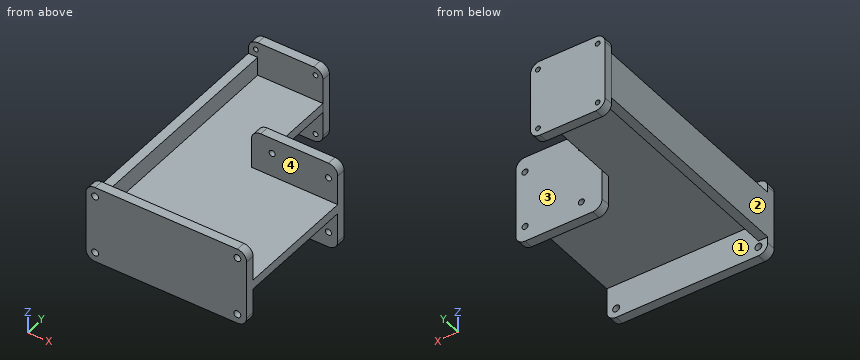
```python
from build123d import *

# Parameters (mm, degrees)
SKT_BASE_W_MOUNTING_HOLES_R           = 1.85
EXT_BASE_PLATE_W_MOUNTING_HOLES_DEPTH = 5
SKT_UPWARD_RIDGE_W                    = 86.25
SKT_UPWARD_RIDGE_H                    = 5
EXT_UPWARD_FLANGE_DEPTH               = 65
EXT_PIX_PLATFORM_DEPTH                = 5
PIX_MOUNT_HOLES_REACH                 = 91.649
SKETCH7_R                             = 1.625
SKETCH8_W                             = 40
SKETCH8_H                             = 5
GPS_FLANGE_DEPTH                      = 55
SKETCH9_R                             = 1.3
GPS_PLATFORM_DEPTH                    = 5
SKETCH10_W                            = 10
SKETCH10_H                            = 120
BRACING_DEPTH                         = 5


with BuildPart() as part:
    # Skt - Base w mounting holes → Ext - Base Plate w Mounting Holes (new body)
    with BuildSketch(Plane(origin=(0, 0, 0), x_dir=(1, 0, 0), z_dir=(0, 1, 0))):
        with BuildLine():
            Line((-38.125, 20.75), (38.125, 20.75))
            ThreePointArc((38.125, 20.75), (41.660533906, 19.285533906), (43.125, 15.75))
            Line((43.125, 15.75), (43.125, -15.75))
            ThreePointArc((43.125, -15.75), (41.660533906, -19.285533906), (38.125, -20.75))
            Line((38.125, -20.75), (-38.125, -20.75))
            ThreePointArc((-38.125, -20.75), (-41.660533906, -19.285533906), (-43.125, -15.75))
            Line((-43.125, -15.75), (-43.125, 15.75))
            ThreePointArc((-43.125, 15.75), (-41.660533906, 19.285533906), (-38.125, 20.75))
        make_face()
        with Locations(Location((-38.125, 15.75, 0), (0, 0, 270))):
            Circle(SKT_BASE_W_MOUNTING_HOLES_R, mode=Mode.SUBTRACT)
        with Locations(Location((38.125, 15.75, 0), (0, 0, 270))):
            Circle(SKT_BASE_W_MOUNTING_HOLES_R, mode=Mode.SUBTRACT)
        with Locations(Location((38.125, -15.75, 0), (0, 0, 270))):
            Circle(SKT_BASE_W_MOUNTING_HOLES_R, mode=Mode.SUBTRACT)
        with Locations(Location((-38.125, -15.75, 0), (0, 0, 270))):
            Circle(SKT_BASE_W_MOUNTING_HOLES_R, mode=Mode.SUBTRACT)
    extrude(amount=EXT_BASE_PLATE_W_MOUNTING_HOLES_DEPTH)

    # Skt - Upward Ridge → Ext - Upward Flange (add)
    with BuildSketch(Plane(origin=(0, 5, 0), x_dir=(1, 0, 0), z_dir=(0, 1, 0))):
        Rectangle(SKT_UPWARD_RIDGE_W, SKT_UPWARD_RIDGE_H)
    extrude(amount=EXT_UPWARD_FLANGE_DEPTH)

    # Skt - GPS Nest → Ext - PIX Platform (add)
    with BuildSketch(Plane(origin=(0, 70, 0), x_dir=(1, 0, 0), z_dir=(0, 1, 0))):
        with BuildLine():
            Line((1.875, 23.5), (38.125, 23.5))
            ThreePointArc((38.125, 23.5), (41.660533906, 22.035533906), (43.125, 18.5))
            Line((43.125, 18.5), (43.125, -18.5))
            ThreePointArc((43.125, -18.5), (41.660533906, -22.035533906), (38.125, -23.5))
            Line((38.125, -23.5), (1.875, -23.5))
            ThreePointArc((1.875, -23.5), (-1.660533906, -22.035533906), (-3.125, -18.5))
            Line((-3.125, -18.5), (-3.125, 18.5))
            ThreePointArc((-3.125, 18.5), (-1.660533906, 22.035533906), (1.875, 23.5))
        make_face()
    extrude(amount=EXT_PIX_PLATFORM_DEPTH)

    # Sketch7 → Pix Mount Holes (cut, up to next)
    with BuildSketch(Plane(origin=(0, 75, 0), x_dir=(1, 0, 0), z_dir=(0, 1, 0)), mode=Mode.PRIVATE) as pix_mount_holes_sk1:
        with Locations(Location((7.975, 15.25, 0), (0, 0, 270))):
            Circle(SKETCH7_R)
    pix_mount_holes_tool1 = extrude(pix_mount_holes_sk1.sketch, amount=-PIX_MOUNT_HOLES_REACH, mode=Mode.PRIVATE) & part.part
    # Sketch7 → Pix Mount Holes (cut, up to next)
    with BuildSketch(Plane(origin=(0, 75, 0), x_dir=(1, 0, 0), z_dir=(0, 1, 0)), mode=Mode.PRIVATE) as pix_mount_holes_sk2:
        with Locations(Location((38.125, 15.25, 0), (0, 0, 270))):
            Circle(SKETCH7_R)
    pix_mount_holes_tool2 = extrude(pix_mount_holes_sk2.sketch, amount=-PIX_MOUNT_HOLES_REACH, mode=Mode.PRIVATE) & part.part
    # Sketch7 → Pix Mount Holes (cut, up to next)
    with BuildSketch(Plane(origin=(0, 75, 0), x_dir=(1, 0, 0), z_dir=(0, 1, 0)), mode=Mode.PRIVATE) as pix_mount_holes_sk3:
        with Locations(Location((38.125, -15.25, 0), (0, 0, 270))):
            Circle(SKETCH7_R)
    pix_mount_holes_tool3 = extrude(pix_mount_holes_sk3.sketch, amount=-PIX_MOUNT_HOLES_REACH, mode=Mode.PRIVATE) & part.part
    # Sketch7 → Pix Mount Holes (cut, up to next)
    with BuildSketch(Plane(origin=(0, 75, 0), x_dir=(1, 0, 0), z_dir=(0, 1, 0)), mode=Mode.PRIVATE) as pix_mount_holes_sk4:
        with Locations(Location((7.975, -15.25, 0), (0, 0, 270))):
            Circle(SKETCH7_R)
    pix_mount_holes_tool4 = extrude(pix_mount_holes_sk4.sketch, amount=-PIX_MOUNT_HOLES_REACH, mode=Mode.PRIVATE) & part.part
    add(pix_mount_holes_tool1.solids().sort_by_distance((7.975, 75, -15.25))[0], mode=Mode.SUBTRACT)
    add(pix_mount_holes_tool2.solids().sort_by_distance((38.125, 75, -15.25))[0], mode=Mode.SUBTRACT)
    add(pix_mount_holes_tool3.solids().sort_by_distance((38.125, 75, 15.25))[0], mode=Mode.SUBTRACT)
    add(pix_mount_holes_tool4.solids().sort_by_distance((7.975, 75, 15.25))[0], mode=Mode.SUBTRACT)

    # Sketch8 → GPS Flange (add)
    with BuildSketch(Plane(origin=(0, 70, 0), x_dir=(1, 0, 0), z_dir=(0, 1, 0))):
        with Locations((-23.125, 0)):
            Rectangle(SKETCH8_W, SKETCH8_H)
    extrude(amount=GPS_FLANGE_DEPTH)

    # Sketch9 → GPS Platform (add)
    with BuildSketch(Plane(origin=(0, 125, 0), x_dir=(1, 0, 0), z_dir=(0, 1, 0))):
        with BuildLine():
            Line((-38.094429072, 20.75), (-8.155570928, 20.75))
            ThreePointArc((-8.155570928, 20.75), (-4.620037022, 19.285533906), (-3.155570928, 15.75))
            Line((-3.155570928, 15.75), (-3.155570928, -15.75))
            ThreePointArc((-3.155570928, -15.75), (-4.620037022, -19.285533906), (-8.155570928, -20.75))
            Line((-8.155570928, -20.75), (-38.094429072, -20.75))
            ThreePointArc((-38.094429072, -20.75), (-41.629962978, -19.285533906), (-43.094429072, -15.75))
            Line((-43.094429072, -15.75), (-43.094429072, 15.75))
            ThreePointArc((-43.094429072, 15.75), (-41.629962978, 19.285533906), (-38.094429072, 20.75))
        make_face()
        with Locations(Location((-39.125, 16.5, 0), (0, 0, 270))):
            Circle(SKETCH9_R, mode=Mode.SUBTRACT)
        with Locations(Location((-7.125, 16.5, 0), (0, 0, 270))):
            Circle(SKETCH9_R, mode=Mode.SUBTRACT)
        with Locations(Location((-7.125, -16.5, 0), (0, 0, 270))):
            Circle(SKETCH9_R, mode=Mode.SUBTRACT)
        with Locations(Location((-39.125, -16.5, 0), (0, 0, 270))):
            Circle(SKETCH9_R, mode=Mode.SUBTRACT)
    extrude(amount=GPS_PLATFORM_DEPTH)

    # Sketch10 → Bracing (add)
    with BuildSketch(Plane.ZY.offset(43.125)):
        with Locations((-7.5, 65)):
            Rectangle(SKETCH10_W, SKETCH10_H)
        with Locations((7.5, 65)):
            Rectangle(SKETCH10_W, SKETCH10_H)
    extrude(amount=-BRACING_DEPTH)


solid = part.part
```
Here's how the part is built. I have some questions about the finished solid (model axes, mm). Face numbers are marked on the shaded views. A direction names the side the tool comes from. Coordinates: 2 decimals unless noted, no trailing zeros. Order: outer loops, then holes, each group sorted by start corner. A loop starts at its lowest first (then second) coordinate and runs counter-clockwise, first axis right, second up.
1) Imagine slicing it at D-D on y = 11. List the corners of the cut face in (x, z) for me (3 decimals).
2) I need wall thicknesses on line 1 (X direction, y = 1.25, z = 15.75) (3 decimals); line 2 (Y direction, x = -8.5, z = 17); line 3 (Y direction, x = 25.5, z = -8). Which ranges of each line are inside material? Lowest first, please.
3) Imagine slicing it at C-C on x = -28. List the corners of the cut face in (y, z) for me.
4) Which directions (+Z, -Z, +X, -X, +Y, -Y) give clear straight access to the entire face, cutting with the end or side of a thin tool? Please do the marked faces 1, 2, 3 and 4.
5) Imagine slicing it at A-A on z = 6. List the corners of the cut face in (x, y) for me (3 decimals), and give its area (3 significant figures).
6) Imagine slicing it at B-B on y = 89. List the corners of the cut face in (x, z) for me (3 decimals).
7) Will these pins go through, and if not, where does the flat tip stop? pin 1 (4 mm diameter, centred on x = -28.5, y = 127.5, fed in from +Z); pin 2 (1.6 mm diameter, centred on x = -7.125, z = 16.5, fed in from +Y); pin 3 (3 mm diameter, centred on x = 15.5, y = 63, fed in from +Z).
Response values:
1. outline: (-43.125, -12.5) - (-38.125, -12.5) - (-38.125, -2.5) - (43.125, -2.5) - (43.125, 2.5) - (-38.125, 2.5) - (-38.125, 12.5) - (-43.125, 12.5) - close
2. line 1: x = -43.125 to -39.975, -36.275 to 36.275, 39.975 to 43.125
2. line 2: y = 0 to 5, 125 to 130
2. line 3: y = 0 to 5, 70 to 75
3. outline: (0, -20.75) - (5, -20.75) - (5, -2.5) - (125, -2.5) - (125, -20.75) - (130, -20.75) - (130, 20.75) - (125, 20.75) - (125, 2.5) - (5, 2.5) - (5, 20.75) - (0, 20.75) - close
4. face 1: -Z, +X
4. face 2: +Z, -Z, -X, +Y, -Y
4. face 3: +Z, -Z, +X, +Y
4. face 4: +Z, +X
5. outline: (-43.125, 0) - (43.125, 0) - (43.125, 5) - (-38.125, 5) - (-38.125, 125) - (-3.156, 125) - (-3.156, 130) - (-43.094, 130) - (-43.094, 125) - (-43.125, 125) - close; (-3.125, 70) - (43.125, 70) - (43.125, 75) - (-3.125, 75) - close
5. area: 1,460 mm2
6. outline: (-43.125, -12.5) - (-38.125, -12.5) - (-38.125, -2.5) - (-3.125, -2.5) - (-3.125, 2.5) - (-38.125, 2.5) - (-38.125, 12.5) - (-43.125, 12.5) - close
7. pin 1: stops at z = 20.75
7. pin 2: stops at y = 5
7. pin 3: stops at z = 2.5
